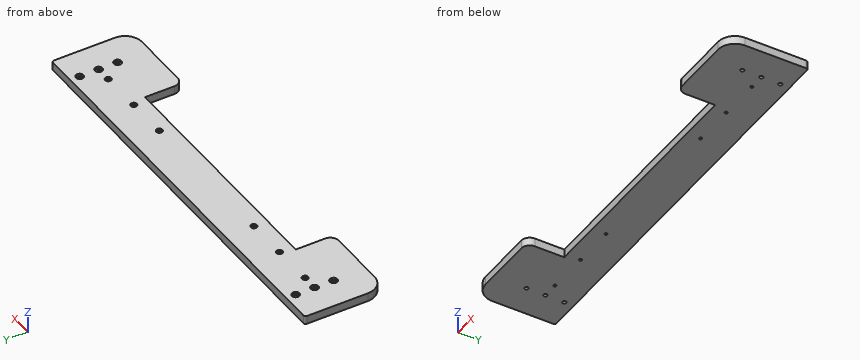
from build123d import *

# Parameters (mm, degrees)
BOSS_EXTRUDE1_DEPTH                    = 20
CBORE_FOR_M8_HEX_HEAD_BOLT1_AT_2_COUNT = 2
CBORE_FOR_M8_HEX_HEAD_BOLT1_AT_2_PITCH = 45
CBORE_FOR_M8_HEX_HEAD_BOLT1_AT_3_COUNT = 2
CBORE_FOR_M8_HEX_HEAD_BOLT1_AT_3_PITCH = 1307.399809271
CBORE_FOR_M8_HEX_HEAD_BOLT1_AT_4_COUNT = 2
CBORE_FOR_M8_HEX_HEAD_BOLT1_AT_4_PITCH = 90
CBORE_FOR_M6_HEX_HEAD_BOLT1_AT_2_COUNT = 2
CBORE_FOR_M6_HEX_HEAD_BOLT1_AT_2_PITCH = 100
CBORE_FOR_M6_HEX_HEAD_BOLT1_AT_3_COUNT = 2
CBORE_FOR_M6_HEX_HEAD_BOLT1_AT_3_PITCH = 200


with BuildPart() as part:
    # Sketch1 → Boss-Extrude1 (new body)
    with BuildSketch(Plane.XY):
        with BuildLine():
            Line((-495, 33.117706736), (-495, 178.117706736))
            ThreePointArc((-495, 178.117706736), (-493.535533906, 181.653240642), (-490, 183.117706736))
            Line((-490, 183.117706736), (490, 183.117706736))
            ThreePointArc((490, 183.117706736), (493.535533906, 181.653240642), (495, 178.117706736))
            Line((495, 178.117706736), (495, 33.117706736))
            ThreePointArc((495, 33.117706736), (483.284271247, 4.833435489), (455, -6.882293264))
            Line((455, -6.882293264), (315, -6.882293264))
            ThreePointArc((315, -6.882293264), (300.857864376, -1.024428888), (295, 13.117706736))
            Line((295, 13.117706736), (295, 83.117706736))
            Line((295, 83.117706736), (-295, 83.117706736))
            Line((-295, 83.117706736), (-295, 13.117706736))
            ThreePointArc((-295, 13.117706736), (-300.857864376, -1.024428888), (-315, -6.882293264))
            Line((-315, -6.882293264), (-455, -6.882293264))
            ThreePointArc((-455, -6.882293264), (-483.284271247, 4.833435489), (-495, 33.117706736))
        make_face()
    extrude(amount=BOSS_EXTRUDE1_DEPTH)

    # Sketch6 → CBORE for M8 Hex Head Bolt1 (revolve, cut)
    with BuildSketch(Plane(origin=(-422.5, 160.617706736, 20), x_dir=(0, -1, 0), z_dir=(1, 0, 0))):
        Polygon((0, 0), (0, 20), (4.5, 20), (4.5, 5.3), (9.0055, 5.3), (9.0055, 0.025), (9.0305, 0), align=None)
    cbore_for_m8_hex_head_bolt1 = revolve(axis=Axis((-422.5, 160.617706736, 26.35), (0, 0, -1)), mode=Mode.SUBTRACT)

    # CBORE for M8 Hex Head Bolt1 at 2: CBORE for M8 Hex Head Bolt1 ×2
    with Locations(*[(0, -i * CBORE_FOR_M8_HEX_HEAD_BOLT1_AT_2_PITCH, 0) for i in range(1, CBORE_FOR_M8_HEX_HEAD_BOLT1_AT_2_COUNT)]):
        add(cbore_for_m8_hex_head_bolt1, mode=Mode.SUBTRACT)

    # CBORE for M8 Hex Head Bolt1 at 3: CBORE for M8 Hex Head Bolt1 ×2
    with Locations(*[Vector(-0.7034023303245859, 0.710791925737724, 0) * (i * CBORE_FOR_M8_HEX_HEAD_BOLT1_AT_3_PITCH) for i in range(1, CBORE_FOR_M8_HEX_HEAD_BOLT1_AT_3_COUNT)]):
        add(cbore_for_m8_hex_head_bolt1, mode=Mode.SUBTRACT)

    # CBORE for M8 Hex Head Bolt1 at 4: CBORE for M8 Hex Head Bolt1 ×2
    with Locations(*[(0, -i * CBORE_FOR_M8_HEX_HEAD_BOLT1_AT_4_PITCH, 0) for i in range(1, CBORE_FOR_M8_HEX_HEAD_BOLT1_AT_4_COUNT)]):
        add(cbore_for_m8_hex_head_bolt1, mode=Mode.SUBTRACT)

    # Mirror1: CBORE for M8 Hex Head Bolt1 across plane
    add(cbore_for_m8_hex_head_bolt1.mirror(Plane(origin=(0, 0, 0), x_dir=(0, 0, 1), z_dir=(1, 0, 0))), mode=Mode.SUBTRACT)

    # Mirror1 copy 1 sketch → Mirror1 copy 1 (revolve, cut)
    with BuildSketch(Plane(origin=(422.5, 115.617706736, 20), x_dir=(0, -1, 0), z_dir=(-1, 0, 0))):
        Polygon((0, 0), (0, -20), (4.5, -20), (4.5, -5.3), (9.0055, -5.3), (9.0055, -0.025), (9.0305, 0), align=None)
    revolve(axis=Axis((422.5, 115.617706736, 26.35), (0, 0, 1)), mode=Mode.SUBTRACT)

    # Mirror1 copy 2 sketch → Mirror1 copy 2 (revolve, cut)
    with BuildSketch(Plane(origin=(1342.128072507, 1089.906934877, 20), x_dir=(0, -1, 0), z_dir=(-1, 0, 0))):
        Polygon((0, 0), (0, -20), (4.5, -20), (4.5, -5.3), (9.0055, -5.3), (9.0055, -0.025), (9.0305, 0), align=None)
    revolve(axis=Axis((1342.128072507, 1089.906934877, 26.35), (0, 0, 1)), mode=Mode.SUBTRACT)

    # Mirror1 copy 3 sketch → Mirror1 copy 3 (revolve, cut)
    with BuildSketch(Plane(origin=(422.5, 70.617706736, 20), x_dir=(0, -1, 0), z_dir=(-1, 0, 0))):
        Polygon((0, 0), (0, -20), (4.5, -20), (4.5, -5.3), (9.0055, -5.3), (9.0055, -0.025), (9.0305, 0), align=None)
    revolve(axis=Axis((422.5, 70.617706736, 26.35), (0, 0, 1)), mode=Mode.SUBTRACT)

    # Sketch8 → CBORE for M6 Hex Head Bolt1 (revolve, cut)
    with BuildSketch(Plane(origin=(-385, 115.617706736, 20), x_dir=(0, -1, 0), z_dir=(1, 0, 0))):
        Polygon((0, 0), (0, 20.001), (3.3, 20.001), (3.3, 4), (7.2735, 4), (7.2735, 0.025), (7.2985, 0), align=None)
    cbore_for_m6_hex_head_bolt1 = revolve(axis=Axis((-385, 115.617706736, 26.35), (0, 0, -1)), mode=Mode.SUBTRACT)

    # CBORE for M6 Hex Head Bolt1 at 2: CBORE for M6 Hex Head Bolt1 ×2
    with Locations(*[(i * CBORE_FOR_M6_HEX_HEAD_BOLT1_AT_2_PITCH, 0, 0) for i in range(1, CBORE_FOR_M6_HEX_HEAD_BOLT1_AT_2_COUNT)]):
        add(cbore_for_m6_hex_head_bolt1, mode=Mode.SUBTRACT)

    # CBORE for M6 Hex Head Bolt1 at 3: CBORE for M6 Hex Head Bolt1 ×2
    with Locations(*[(i * CBORE_FOR_M6_HEX_HEAD_BOLT1_AT_3_PITCH, 0, 0) for i in range(1, CBORE_FOR_M6_HEX_HEAD_BOLT1_AT_3_COUNT)]):
        add(cbore_for_m6_hex_head_bolt1, mode=Mode.SUBTRACT)

    # Mirror2: CBORE for M6 Hex Head Bolt1 across plane
    add(cbore_for_m6_hex_head_bolt1.mirror(Plane(origin=(0, 0, 0), x_dir=(0, 0, 1), z_dir=(1, 0, 0))), mode=Mode.SUBTRACT)

    # Mirror2 copy 1 sketch → Mirror2 copy 1 (revolve, cut)
    with BuildSketch(Plane(origin=(285, 115.617706736, 20), x_dir=(0, -1, 0), z_dir=(-1, 0, 0))):
        Polygon((0, 0), (0, -20.001), (3.3, -20.001), (3.3, -4), (7.2735, -4), (7.2735, -0.025), (7.2985, 0), align=None)
    revolve(axis=Axis((285, 115.617706736, 26.35), (0, 0, 1)), mode=Mode.SUBTRACT)

    # Mirror2 copy 2 sketch → Mirror2 copy 2 (revolve, cut)
    with BuildSketch(Plane(origin=(185, 115.617706736, 20), x_dir=(0, -1, 0), z_dir=(-1, 0, 0))):
        Polygon((0, 0), (0, -20.001), (3.3, -20.001), (3.3, -4), (7.2735, -4), (7.2735, -0.025), (7.2985, 0), align=None)
    revolve(axis=Axis((185, 115.617706736, 26.35), (0, 0, 1)), mode=Mode.SUBTRACT)


solid = part.part
The model under review builds one solid part; all positions refer to its coordinate system, in mm. Coordinates: 2 decimals unless noted, no trailing zeros. Loops run counter-clockwise (first coordinate to the right, second up) from the corner with the lowest first, then second, coordinate; pieces in that order, holes last. Notation, with made-up numbers: M 21.25,13 L 50.25,13 A29 ccw 50.25,38 Z; hole C -23,-0.5 d3. An arc over 180 degrees is marked long. Put each result on its own line as item: value. Start each with the question number.
Q1. Add section C-C (x = -148.5). Write out the cut boundary in (y, z).
Q2. Add section B-B (z = 8.75). Count the separate pieces of the cut face and the enclosed holes in it, and give its area (3 significant figures).
Q3. Add section A-A (y = 42). Write out the cut boundary in (x, z).
Q4. Clearance check with flat-ended pins moving along their axes: pin 1 (7.5 mm diameter, centred on x = 185, y = 118.5, fed in from +Z); pin 2 (16 mm diameter, centred on x = 422.5, y = 70.62, fed in from +Z). State where each tip first meets the part, or that it passes through.
Q5. Wall thickness on line 1 (Y direction, x = 422.5, z = 6.25); line 2 (X direction, y = 61, z = 6); line 3 (X direction, y = 160, z = 15.5): over which ranges is each line inside the solid? List them lowest first.
Answers:
1. outline: M 83.12,0 L 183.12,0 L 183.12,20 L 83.12,20 Z
2. separate pieces: 1
2. enclosed holes: 12
2. area: 134,000 mm^2
3. outline: M -495,0 L -295,0 L -295,20 L -495,20 Z; M 295,0 L 495,0 L 495,20 L 295,20 Z
4. pin 1: stops at z = 16
4. pin 2: stops at z = 14.7
5. line 1: y = -6.88 to 66.12, 75.12 to 111.12, 120.12 to 156.12, 165.12 to 183.12
5. line 2: x = -495 to -295, 295 to 495
5. line 3: x = -495 to -431.48, -413.52 to 413.52, 431.48 to 495
